The model under review builds one solid part; all positions refer to its coordinate system, in mm. A direction names the side the tool comes from. Coordinates: 2 decimals unless noted, no trailing zeros. Write each loop counter-clockwise with the first axis right and the second up, starting at its lowest first coordinate (ties: lowest second). Pieces come first, ordered by that corner, then holes. Notation, with made-up numbers: (67, 74) -> (118, 74) arc R21 cw to (118, 96) -> close; hole circle Ø2 at (60, 5). An arc over 180 degrees is marked (long way). Write each question's results on one line, items separated by ' | '.
```python
from build123d import *

# Parameters (mm, degrees)
SKETCH1_W           = 40.7
SKETCH1_H           = 20
BOSS_EXTRUDE1_DEPTH = 8
SKETCH2_R           = 2.35
CUT_EXTRUDE1_DEPTH  = 10
CUT_EXTRUDE2_START  = -10
SKETCH3_R           = 2.35
CUT_EXTRUDE2_DEPTH  = 10
CHAMFER1_SIZE       = 1


with BuildPart() as part:
    # Sketch1 → Boss-Extrude1 (new body)
    with BuildSketch(Plane(origin=(0, 0, 0), x_dir=(1, 0, 0), z_dir=(0, 1, 0))):
        Rectangle(SKETCH1_W, SKETCH1_H)
    extrude(amount=BOSS_EXTRUDE1_DEPTH)

    # Sketch2 → Cut-Extrude1 (cut)
    with BuildSketch(Plane(origin=(20.35, 0, 0), x_dir=(0, 0, -1), z_dir=(1, 0, 0))):
        with Locations((0, 4)):
            Circle(SKETCH2_R)
    extrude(amount=-CUT_EXTRUDE1_DEPTH, mode=Mode.SUBTRACT)

    # Sketch3 → Cut-Extrude2 (cut)
    with BuildSketch(Plane.ZY.offset(20.35).offset(CUT_EXTRUDE2_START)):
        with Locations(Location((0, 4, 0), (0, 0, 180))):
            Circle(SKETCH3_R)
    extrude(amount=CUT_EXTRUDE2_DEPTH, mode=Mode.SUBTRACT)

    # Chamfer1
    chamfer1_edges = [part.edges().sort_by_distance(p)[0] for p in [
        (20.35, 4, 2.35),
        (-20.35, 4, 2.35),
    ]]
    chamfer(chamfer1_edges, length=CHAMFER1_SIZE)


solid = part.part
```
Q1. Add section A-A (y = 4). Write out the cut boundary in (x, z), plus the area to 3 significant figures.
Solution:
outline: (-20.35, -10) -> (20.35, -10) -> (20.35, -3.35) -> (19.35, -2.35) -> (10.35, -2.35) -> (10.35, 2.35) -> (19.35, 2.35) -> (20.35, 3.35) -> (20.35, 10) -> (-20.35, 10) -> (-20.35, 3.35) -> (-19.35, 2.35) -> (-10.35, 2.35) -> (-10.35, -2.35) -> (-19.35, -2.35) -> (-20.35, -3.35) -> close | area: 718 mm²
Q2. Add section B-B (z = 0). Write out the cut boundary in (x, y).
Solution:
outline: (-20.35, 0) -> (20.35, 0) -> (20.35, 0.65) -> (19.35, 1.65) -> (10.35, 1.65) -> (10.35, 6.35) -> (19.35, 6.35) -> (20.35, 7.35) -> (20.35, 8) -> (-20.35, 8) -> (-20.35, 7.35) -> (-19.35, 6.35) -> (-10.35, 6.35) -> (-10.35, 1.65) -> (-19.35, 1.65) -> (-20.35, 0.65) -> close
Q3. Draft analysis for pull direction Z (two halves, no side actions). For faces 4 (the flat face through (-20.35, 1, 2)), 5 (the cylindrical face through (14.91, 4.71, -2.24)), 6 (the flat face through (0, 4, 10)), state which applies: pulls with the +Z half, pulls with the -Z half, needs draft (parallel to the pull), parting line crosses it, or undercut.
Solution:
face 4: needs draft | face 5: undercut | face 6: pulls with the +Z half
Q4. Machinability: for faces 1 (the flat face through (10.35, 4, 0)), 2 (the flat face through (0, 8, 0)), 3 (the flat face through (-10.35, 4, 0)), which of the approach directions +Z, -Z, +X, -X, +Y, -Y give a long, thin tool a straight path to every point of the face, cutting with its end or side? Answer none if there is none.
Solution:
face 1: +X | face 2: +Z, -Z, +X, -X, +Y | face 3: -X
Q5. For line 1 (Y direction, x = -15.25, z = 0); line 2 (Z direction, x = -15.5, y = 4); line 3 (X direction, y = 4.25, z = -0.25), list the stretches that pass through material, from the lowest coordinate up. Write a range as from..to.
Solution:
line 1: 0..1.65, 6.35..8 | line 2: -10..-2.35, 2.35..10 | line 3: -10.35..10.35
